Input: dimensioned drawing with shaded views. Units: mm. Origin: part minimum x, y, z. A direction names the side the tool comes from. Round coordinates to 2 decimals unless told otherwise and drop trailing zeros. Order: outer loops, then holes, each group sorted by start corner. A loop starts at its lowest first (then second) coordinate and runs counter-clockwise, first axis right, second up. Notation, with made-up numbers: M -27,-15 L 22,-15 A22 cw 22,3 Z; hole C 63.5,26.25 d8. An arc over 180 degrees is marked long. One line per question, with ' | ' between items.
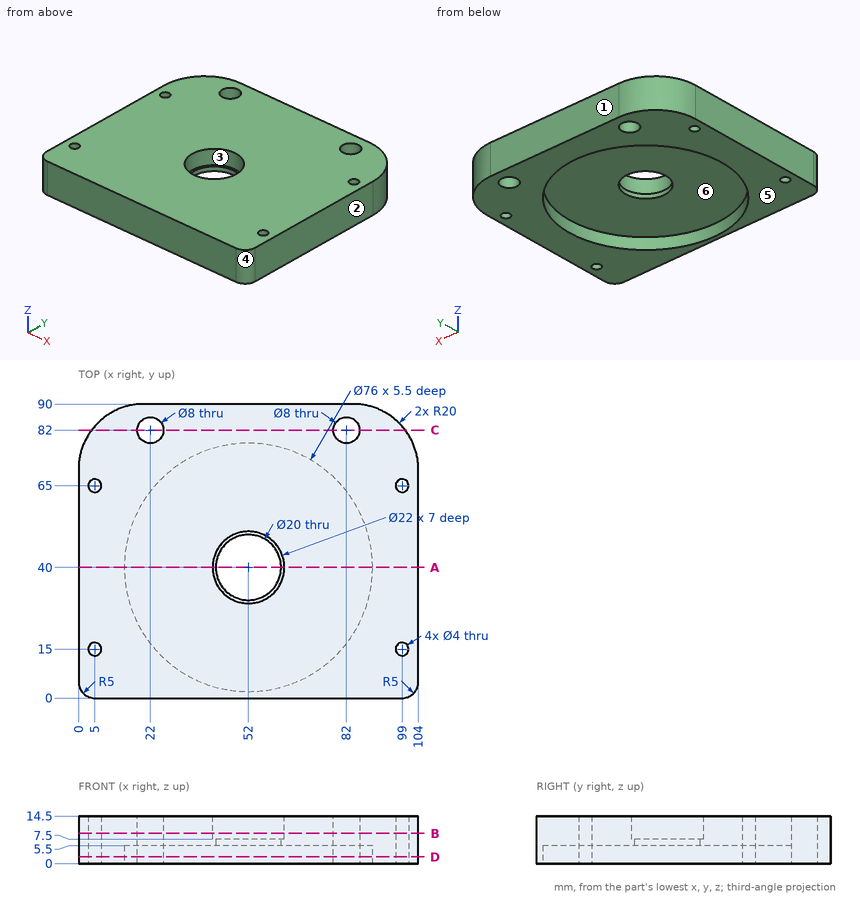
Item 1: Line query: line 1 along X through (y, z) = (83, 9); line 2 along Y through (x, z) = (52, 6.1); line 3 along Z through (x, y) = (53, 15). Output: solid intervals per line, ascending. Write a range as from..to.
Report:
line 1: 4.8..18.13, 25.87..78.13, 85.87..99.2 | line 2: 0..30, 50..90 | line 3: 5.5..14.5
Item 2: Section query A-A, the plane y = 40. Return loops of the section in (x, z).
Report:
outline: M 0,0 L 14,0 L 14,5.5 L 42,5.5 L 42,7.5 L 41,7.5 L 41,14.5 L 0,14.5 Z; M 62,5.5 L 90,5.5 L 90,0 L 104,0 L 104,14.5 L 63,14.5 L 63,7.5 L 62,7.5 Z
Item 3: Section query D-D, the plane z = 2. Return loops of the section in (x, y).
Report:
outline: M 0,5 A5 ccw 5,0 L 99,0 A5 ccw 104,5 L 104,70 A20 ccw 84,90 L 20,90 A20 ccw 0,70 Z; hole C 5,15 d4; hole C 5,65 d4; hole C 52,40 d76; hole C 22,82 d8; hole C 82,82 d8; hole C 99,15 d4; hole C 99,65 d4
Item 4: Section query B-B, the plane z = 9.25. Return loops of the section in (x, y), plus the area to 3 significant figures.
Report:
outline: M 0,5 A5 ccw 5,0 L 99,0 A5 ccw 104,5 L 104,70 A20 ccw 84,90 L 20,90 A20 ccw 0,70 Z; hole C 5,15 d4; hole C 5,65 d4; hole C 22,82 d8; hole C 52,40 d22; hole C 82,82 d8; hole C 99,15 d4; hole C 99,65 d4 | area: 8,650 mm²
Item 5: Section query C-C, the plane y = 82. Return loops of the section in (x, z).
Report:
outline: M 4,0 L 18,0 L 18,14.5 L 4,14.5 Z; M 26,0 L 78,0 L 78,14.5 L 26,14.5 Z; M 86,0 L 100,0 L 100,14.5 L 86,14.5 Z
Item 6: Access query for the marked faces 5 and 6. Directions: +Z, -Z, +X, -X, +Y, -Y. A direction counts if a zero-diameter tool reaches every point of the face in a straight line with its end or side. Return the directions, or none.
Report:
face 5: -Z, +X, -X, +Y, -Y | face 6: -Z
Item 7: First-contact query: pin 1 (3 mm diameter, centred on x = 64, y = 20, fed in from -Z). Flat tip, straight axial feed; report the tip coordinate or a pass-through.
Report:
pin 1: z = 5.5
Item 8: Mould query, pull axis Y, two halves, no side actions, for the marked faces 1, 2, 3 and 4. Classes: +Y half, -Y half, draft (parallel to the pull), parting line (faces both ways), or undercut.
Report:
face 1: +Y half | face 2: draft | face 3: undercut | face 4: -Y half
